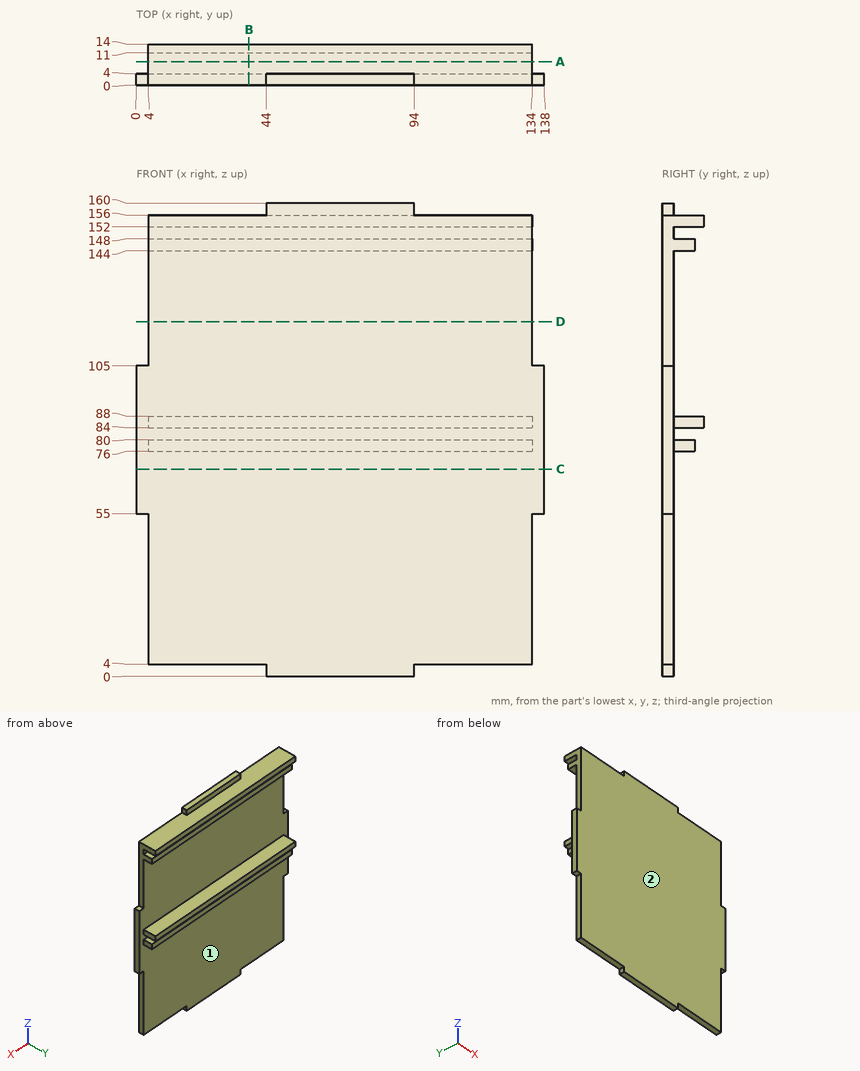
Here's the drawing with two shaded views (mm, measured from the low corner). I have some questions. Coordinates: 2 decimals unless noted, no trailing zeros. Order: outer loops, then holes, each group sorted by start corner. A loop starts at its lowest first (then second) coordinate and runs counter-clockwise, first axis right, second up. Notation, with made-up numbers: (89, 86.25) - (103, 86.25) arc R15 cw to (103, 99.25) - close; hole circle Ø5 at (11, 55.5). An arc over 180 degrees is marked (long way). Use CSV: the item, a comma, the result in double quotes. Start each with the question number.
1. Please list where these lines run through material, in increasing order: line 1 (Z direction, x = 90, y = 4.5); line 2 (Z direction, x = 62, y = 13); line 3 (Z direction, x = 42.5, y = 2.5). Write a range as from..to.
2. Suppose I cut it at D-D on z = 120. List the corners of the cut face in (x, y) for me.
3. If we mould it in two halves opening along Z, with no side actions, what happens to the marked faces 1 and 2? For each: +Z half, -Z half, draft (parallel to the pull), parting line (faces both ways), or undercut.
4. Suppose I cut it at A-A on y = 8. List the corners of the cut face in (x, z) for me, then the cut area to 3 significant figures.
5. Suppose I cut it at B-B on x = 38. List the corners of the cut face in (y, z) for me.
6. I'm going to push flat-ended pins straight in: pin 1 (5 mm diameter, centred on x = 117, y = 5.5, fed in from -Z); pin 2 (3 mm diameter, centred on y = 7.5, z = 85.5, fed in from +X); pin 3 (3 mm diameter, centred on x = 58.5, z = 77.5, fed in from +Y). Where does each tip first touch, or does it pass through?
7. Suppose I cut it at C-C on z = 70. List the corners of the cut face in (x, y) for me.
Output:
1,line 1,"z = 76..80, 84..88, 144..148, 152..156"
1,line 2,"z = 84..88, 152..156"
1,line 3,"z = 4..156"
2,outline,"(4, 0) - (134, 0) - (134, 4) - (4, 4) - close"
3,face 1,"undercut"
3,face 2,"draft"
4,outline,"(4, 76) - (134, 76) - (134, 80) - (4, 80) - close; (4, 84) - (134, 84) - (134, 88) - (4, 88) - close; (4, 144) - (134, 144) - (134, 148) - (4, 148) - close; (4, 152) - (134, 152) - (134, 156) - (4, 156) - close"
4,area,"2,080 mm2"
5,outline,"(0, 4) - (4, 4) - (4, 76) - (11, 76) - (11, 80) - (4, 80) - (4, 84) - (14, 84) - (14, 88) - (4, 88) - (4, 144) - (11, 144) - (11, 148) - (4, 148) - (4, 152) - (14, 152) - (14, 156) - (0, 156) - close"
6,pin 1,"stops at z = 4"
6,pin 2,"stops at x = 134"
6,pin 3,"stops at y = 11"
7,outline,"(0, 0) - (138, 0) - (138, 4) - (0, 4) - close"
